from build123d import *

# Parameters (mm, degrees)
BOSS_EXTRU_1_DEPTH = 10.5
D_GAGEMENT_M41_D   = 4.8


with BuildPart() as part:
    # Esquisse1 → Boss.-Extru.1 (new body)
    with BuildSketch(Plane(origin=(0, 0, 0), x_dir=(1, 0, 0), z_dir=(0, 1, 0))):
        with BuildLine():
            Line((0, 0), (12, 0))
            ThreePointArc((12, 0), (12.591460154, 0.325600632), (12.632692308, 0.999500324))
            ThreePointArc((12.632692308, 0.999500324), (16.7, 7.424859546), (20.767307692, 0.999500324))
            ThreePointArc((20.767307692, 0.999500324), (20.808539846, 0.325600632), (21.4, 0))
            Line((21.4, 0), (22.056304696, 0))
            ThreePointArc((22.056304696, 0), (22.444916153, 0.117779135), (22.702755263, 0.431482469))
            ThreePointArc((22.702755263, 0.431482469), (17.871531541, 9.318412068), (10.20317064, 2.721861345))
            ThreePointArc((10.20317064, 2.721861345), (10.006156571, 2.212815713), (9.503512094, 2))
            Line((9.503512094, 2), (0, 2))
            ThreePointArc((0, 2), (-0.494974747, 1.794974747), (-0.7, 1.3))
            Line((-0.7, 1.3), (-0.7, 0.7))
            ThreePointArc((-0.7, 0.7), (-0.494974747, 0.205025253), (0, 0))
        make_face()
    extrude(amount=BOSS_EXTRU_1_DEPTH)

    # Dégagement M41 (through all)
    with Locations(Plane(origin=(0, 0, -2), x_dir=(-1, 0, 0), z_dir=(0, 0, -1))):
        with Locations((-4.751756047, 5.25)):
            Hole(D_GAGEMENT_M41_D / 2)


solid = part.part
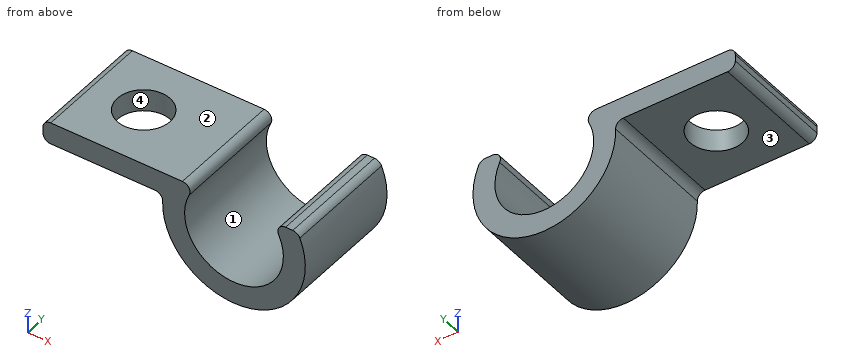
Input: part model. Units: mm. Frame: model coordinates. Face numbers are marked on the shaded views. Coordinates: 2 decimals unless noted, no trailing zeros. Loops run counter-clockwise (first coordinate to the right, second up) from the corner with the lowest first, then second, coordinate; pieces in that order, holes last.
(1) Section C-C on z = -5.25. Return the cut outline in (x, y), then the cut area to 3 significant figures.
(2) Section A-A on y = 6. Return the cut outline in (x, z), then the cut area to 3 significant figures.
(3) Section B-B on x = 3.25. Return the cut outline in (y, z).
(4) First-contact query: pin 1 Ø1.5 at (x, y) = (3.5, 6.5) entering from -Z. Flat tip, straight axial feed; report the tip coordinate or a pass-through.
(5) Pull-direction query (Z, two-part tool) for the marked faces 1, 2, 3 and 4; classes: released by +Z, released by -Z, zero draft, split by the parting line, or undercut.
(6) Section D-D on y = 9.25. Return the cut outline in (x, z), then the cut area to 3 significant figures.
(7) Material intervals for probe 1 along X at (y, z) = (1.5, -3); probe 2 along X at (y, z) = (0.5, -1); probe 3 along Z at (x, y) = (7.25, 8.75), sorted ascending.
Data:
1. outline: (10.63, 0) - (12.85, 0) - (12.85, 10.5) - (10.63, 10.5) - close; (20.55, 0) - (22.77, 0) - (22.77, 10.5) - (20.55, 10.5) - close
1. area: 46.6 mm2
2. outline: (-0.7, -1.3) arc R0.7 ccw to (0, -2) - (2.47, -2) - (2.47, 0) - (0, 0) arc R0.7 ccw to (-0.7, -0.7) - close; (7.03, -2) - (9.5, -2) arc R0.7 cw to (10.2, -2.72) arc R6.5 ccw (long way) to (22.7, -0.43) arc R0.7 ccw to (22.06, 0) - (21.4, 0) arc R0.7 ccw to (20.77, -1) arc R4.5 cw (long way) to (12.63, -1) arc R0.7 ccw to (12, 0) - (7.03, 0) - close
2. area: 59.5 mm2
3. outline: (0, -2) - (3.38, -2) - (3.38, 0) - (0, 0) - close; (7.12, -2) - (10.5, -2) - (10.5, 0) - (7.12, 0) - close
4. pin 1: stops at z = -2
5. face 1: undercut
5. face 2: released by +Z
5. face 3: released by -Z
5. face 4: zero draft
6. outline: (-0.7, -1.3) arc R0.7 ccw to (0, -2) - (9.5, -2) arc R0.7 cw to (10.2, -2.72) arc R6.5 ccw (long way) to (22.7, -0.43) arc R0.7 ccw to (22.06, 0) - (21.4, 0) arc R0.7 ccw to (20.77, -1) arc R4.5 cw (long way) to (12.63, -1) arc R0.7 ccw to (12, 0) - (0, 0) arc R0.7 ccw to (-0.7, -0.7) - close
6. area: 68.6 mm2
7. probe 1: x = 10.2 to 12.2, 21.2 to 23.2
7. probe 2: x = -0.7 to 12.63, 20.77 to 22.91
7. probe 3: z = -2 to 0
